The model under review builds one solid part; all positions refer to its coordinate system, in mm. A direction names the side the tool comes from. Round coordinates to 2 decimals unless told otherwise and drop trailing zeros. Order: outer loops, then holes, each group sorted by start corner. A loop starts at its lowest first (then second) coordinate and runs counter-clockwise, first axis right, second up. Notation, with made-up numbers: M -30,12 L 21,12 A22 cw 21,42 Z; hole C 23,25.25 d2. An arc over 180 degrees is marked long. Answer as a JSON object with one key per item and string values. Group by question number.
1) To check wall thickness, follow line 1 (X direction, y = 3.4, z = 15); line 2 (X direction, y = 3.7, z = 2); line 3 (Z direction, x = -54, y = 1.4). State the ranges of each line that lie inside material, in increasing order.
2) Consider section B-B, the plane x = -3.5. Write out the cut boundary in (y, z).
3) For faces 4 (the flat face through (-42.5, 2, -33)), 5 (the flat face through (-16, 5, 0)), 6 (the flat face through (0, 2, 33)), 7 (the flat face through (-2.5, 2, 1)), list the 3-axis set-ups (+Z, -Z, +X, -X, +Y, -Y) from which the entire face can be reached by the end or side of a thin tool; tool diameter is ignored.
4) Consider section C-C, the plane z = -11.5. Write out the cut boundary in (x, y), then the cut area to 4 significant figures.
5) The part is to be moulded in two halves that separate along X. For faces 1 (the flat face through (-14, 2, 30)), 2 (the flat face through (-57.5, 2, 0)), 3 (the flat face through (15, 2, -33)), say which applies: +X half, -X half, draft (parallel to the pull), parting line (faces both ways), or undercut.
6) Insertion check: pin 1 Ø1.5 at (x, y) = (-52, 2) entering from +Z; pin 2 Ø2.5 at (x, y) = (-5, 3) entering from -Z. Each pin has a flat end and moves straight along its axis. Give the tip position at first contact, or say it passes through.
7) Consider section A-A, the plane z = 15. Write out the cut boundary in (x, y), then the cut area to 4 significant figures.
8) Consider section D-D, the plane x = -18.5. Write out the cut boundary in (y, z).
```python
from build123d import *

# Parameters (mm, degrees)
SKETCH1_R           = 8
SKETCH1_W           = 10
SKETCH1_H           = 5.2
SKETCH1_W_2         = 5.2
SKETCH1_H_2         = 12
BOSS_EXTRUDE1_DEPTH = 5


with BuildPart() as part:
    # Sketch1 → Boss-Extrude1 (new body)
    with BuildSketch(Plane(origin=(0, 0, 0), x_dir=(1, 0, 0), z_dir=(0, 1, 0))):
        Polygon((25, 30), (25, -30), (15, -30), (15, -35.1), (0, -35.1), (0, -30), (-27.5, -30), (-27.5, -35.1), (-42.5, -35.1), (-42.5, -30), (-57.5, -30), (-57.5, 30), (-42.5, 30), (-42.5, 35.1), (-27.5, 35.1), (-27.5, 30), (0, 30), (0, 35.1), (15, 35.1), (15, 30), align=None)
        with Locations(Location((-27.5, -15, 0), (0, 0, 270))):
            Circle(SKETCH1_R, mode=Mode.SUBTRACT)
        with Locations(Location((-3.5, -15, 0), (0, 0, 270))):
            Circle(SKETCH1_R, mode=Mode.SUBTRACT)
        with Locations((-22.5, -1.4)):
            Rectangle(SKETCH1_W, SKETCH1_H, mode=Mode.SUBTRACT)
        with Locations((-7.5, -1.4)):
            Rectangle(SKETCH1_W, SKETCH1_H, mode=Mode.SUBTRACT)
        with Locations((-51.9, -12)):
            Rectangle(SKETCH1_W_2, SKETCH1_H_2, mode=Mode.SUBTRACT)
        with Locations((-51.9, 12)):
            Rectangle(SKETCH1_W_2, SKETCH1_H_2, mode=Mode.SUBTRACT)
    extrude(amount=BOSS_EXTRUDE1_DEPTH)


solid = part.part
```
Results list:
{
 "1": {"line 1": "-57.5 to -54.5, -49.3 to -35.5, -19.5 to -11.5, 4.5 to 25", "line 2": "-57.5 to -27.5, -17.5 to -12.5, -2.5 to 25", "line 3": "-30 to -18, -6 to 6, 18 to 30"},
 "2": {"outline": "M 0,-30 L 5,-30 L 5,-1.2 L 0,-1.2 Z; M 0,4 L 5,4 L 5,7 L 0,7 Z; M 0,23 L 5,23 L 5,30 L 0,30 Z"},
 "3": {"face 4": "-Z, -X, +Y, -Y", "face 5": "+Z, -Z, +X, -X, +Y", "face 6": "+Z, +Y, -Y", "face 7": "+Y, -Y"},
 "4": {"outline": "M -57.5,0 L -54.5,0 L -54.5,5 L -57.5,5 Z; M -49.3,0 L 25,0 L 25,5 L -49.3,5 Z", "area": "386.5 mm^2"},
 "5": {"face 1": "undercut", "face 2": "-X half", "face 3": "+X half"},
 "6": {"pin 1": "z = 30", "pin 2": "z = -30"},
 "7": {"outline": "M -57.5,0 L -54.5,0 L -54.5,5 L -57.5,5 Z; M -49.3,0 L -35.5,0 L -35.5,5 L -49.3,5 Z; M -19.5,0 L -11.5,0 L -11.5,5 L -19.5,5 Z; M 4.5,0 L 25,0 L 25,5 L 4.5,5 Z", "area": "226.5 mm^2"},
 "8": {"outline": "M 0,-30 L 5,-30 L 5,-1.2 L 0,-1.2 Z; M 0,4 L 5,4 L 5,30 L 0,30 Z"}
}
